Input: part model. Units: mm. Frame: model coordinates. A direction names the side the tool comes from. Coordinates: 2 decimals unless noted, no trailing zeros. Order: outer loops, then holes, each group sorted by start corner. A loop starts at its lowest first (then second) coordinate and runs counter-clockwise, first axis right, second up. Notation, with made-up numbers: (59.5, -32.5) - (65.5, -32.5) arc R15 ccw to (65.5, -24.5) - close; hole circle Ø5 at (-34.75, 69). An arc over 180 degrees is marked (long way). One line per question, with ' | ' between items.
from build123d import *

# Parameters (mm, degrees)
F1_DEPTH       = 12.7
F3_D           = 6.7564
F3_CSINK_D     = 13.4874
F3_CSINK_ANGLE = 82
F5_D           = 6.7564
F5_CSINK_D     = 13.4874
F5_CSINK_ANGLE = 82
F6_R           = 3.175
F7_R           = 9.525
F8_R           = 1.524


with BuildPart() as f1:
    # F0 (on Right) → F1 (new body, symmetric)
    with BuildSketch(Plane.YZ):
        Polygon((-36.0811725259, 16.0017143935), (-36.0811725259, 9.6517140046), (59.1688280165, 9.6517140046), (59.1688280165, -85.5982856065), (65.5188274741, -85.5982856065), (65.5188274741, 16.0017143935), align=None)
    extrude(amount=F1_DEPTH, both=True)

    # F3 (through all)
    with Locations(Plane.XZ.offset(-59.1688280165)):
        with Locations((0, -9.3982859954), (0, -60.1982859954)):
            CounterSinkHole(F3_D / 2, F3_CSINK_D / 2, counter_sink_angle=F3_CSINK_ANGLE)

    # F5 (through all)
    with Locations(Plane(origin=(0, 0, 9.6517140046), x_dir=(1, 0, 0), z_dir=(0, 0, -1))):
        with Locations((0, 10.6811719835), (0, -40.1188280165)):
            CounterSinkHole(F5_D / 2, F5_CSINK_D / 2, counter_sink_angle=F5_CSINK_ANGLE)

    # F6
    f6_edges = [f1.edges().sort_by_distance(p)[0] for p in [
        (0, 59.168828, 9.651714),
    ]]
    fillet(f6_edges, radius=F6_R)

    # F7
    f7_edges = [f1.edges().sort_by_distance(p)[0] for p in [
        (0, 65.518827, 16.001714),
    ]]
    fillet(f7_edges, radius=F7_R)

    # F8
    f8_edges = [f1.edges().sort_by_distance(p)[0] for p in [
        (12.7, 62.343828, -85.598286),
        (12.7, -36.081173, 12.826714),
        (-12.7, -36.081173, 12.826714),
        (-12.7, 62.343828, -85.598286),
        (0, 65.518827, -85.598286),
        (0, -36.081173, 16.001714),
        (0, -36.081173, 9.651714),
        (0, 59.168828, -85.598286),
    ]]
    fillet(f8_edges, radius=F8_R)


solid = f1.part
Item 1: Access query for faces 1 (the face through (0, 10, 9.652)), 2 (the face through (0, 62, -85.598)). Directions: +Z, -Z, +X, -X, +Y, -Y. A direction counts if a zero-diameter tool reaches every point of the face in a straight line with its end or side. Return the directions, or none.
Data:
face 1: -Z, +X, -X, -Y | face 2: -Z, +X, -X, +Y, -Y
Item 2: Section D-D on y = 58. Return the cut outline in (x, z), and give its area (3 significant figures).
Data:
outline: (-12.7, 8.94) - (12.7, 8.94) - (12.7, 15.79) - (-12.7, 15.79) - close | area: 174 mm^2
Item 3: Section B-B on x = 0. Count the separate pieces of the cut face and the enclosed holes in it, and give its area (3 significant figures).
Data:
separate pieces: 5 | enclosed holes: 0 | area: 1,010 mm^2
Item 4: Contact query for flat-ended pins moving along their axis: P1, Ø12.5, axis at x = 6.5, z = -61, coming from the -Y side; P2, Ø8, axis at x = 1, y = 24, coming from the -Z side. Output: stop coordinate, or through.
Data:
P1: y = 59.17 | P2: z = 9.65
Item 5: Ray query, line 1 (Z direction, x = 0, y = 63.9); line 2 (Y direction, x = 4.5, z = -24); line 3 (Y direction, x = 0, z = 14.15). Return the intervals inside material, ascending.
Data:
line 1: -85.6 to -63.58, -56.82 to -12.78, -6.02 to 11.79 | line 2: 59.17 to 65.52 | line 3: -36.08 to -14.06, -7.3 to 36.74, 43.5 to 61.64
Item 6: Section A-A on x = -9. Return the cut outline in (y, z) (3 decimals).
Data:
outline: (-36.081, 11.176) arc R1.524 ccw to (-34.557, 9.652) - (55.994, 9.652) arc R3.175 cw to (59.169, 6.477) - (59.169, -84.074) arc R1.524 ccw to (60.693, -85.598) - (63.995, -85.598) arc R1.524 ccw to (65.519, -84.074) - (65.519, 6.477) arc R9.525 ccw to (55.994, 16.002) - (-34.557, 16.002) arc R1.524 ccw to (-36.081, 14.478) - close
Item 7: Draft query along X for faces 3 (the face through (0.18, 58.26, 8.7)), 4 (the face through (12.7, 37, 11)), 5 (the face through (0.77, 62.85, -63.66)). Return one class per face: released by +X, released by -X, zero draft, split by the parting line, or undercut.
Data:
face 3: zero draft | face 4: released by +X | face 5: undercut
Item 8: Section C-C on z = -45. Return the cut outline in (x, y), and give its area (3 significant figures).
Data:
outline: (-12.7, 59.17) - (12.7, 59.17) - (12.7, 65.52) - (-12.7, 65.52) - close | area: 161 mm^2
